The model under review builds one solid part; all positions refer to its coordinate system, in mm. Coordinates: 2 decimals unless noted, no trailing zeros. Order: outer loops, then holes, each group sorted by start corner. A loop starts at its lowest first (then second) coordinate and runs counter-clockwise, first axis right, second up.
from build123d import *

# Parameters (mm, degrees)
SKETCH_1_W      = 20
SKETCH_1_H      = 40
SKETCH_1_R      = 4.5
EXTRUDE_1_DEPTH = 47.5
CHAMFER_1_SIZE  = 2
CHAMFER_2_SIZE  = 2


with BuildPart() as part:
    # 草图1 → 凸台-拉伸1 (new body)
    with BuildSketch(Plane.XY):
        Rectangle(SKETCH_1_W, SKETCH_1_H)
        with Locations((0, 10)):
            Circle(SKETCH_1_R, mode=Mode.SUBTRACT)
        with Locations((0, -10)):
            Circle(SKETCH_1_R, mode=Mode.SUBTRACT)
    extrude(amount=EXTRUDE_1_DEPTH)

    # 倒角1
    chamfer_1_edges = [part.edges().sort_by_distance(p)[0] for p in [
        (-10, -20, 23.75),
    ]]
    chamfer(chamfer_1_edges, length=CHAMFER_1_SIZE)

    # 倒角2
    chamfer_2_edges = [part.edges().sort_by_distance(p)[0] for p in [
        (10, -20, 23.75),
        (-10, 20, 23.75),
        (10, 20, 23.75),
    ]]
    chamfer(chamfer_2_edges, length=CHAMFER_2_SIZE)


solid = part.part
(1) Insertion check: pin 1 Ø7 at (x, y) = (0, -10) entering from +Z. The pin has a flat end and moves straight along its axis. Give the tip position at first contact, or say it passes through.
(2) Consider section A-A (y = -10). Give the boundary of the cut face in (x, z).
(3) Consider section C-C (z = 6.5). Give the boundary of the cut face in (x, y).
(4) Wall thickness on line 1 (Y direction, x = 0, z = 10); line 2 (Y direction, x = 3.5, z = 40.5); line 3 (X direction, y = 14, z = 40.5): over which ranges is each line inside the solid? List them lowest first.
(5) The part is to be moulded in two halves that separate along Y. For faces 1 (the face through (9, -19, 23)), 2 (the face through (-0.98, -14.39, 23.42)), 3 (the face through (0, 0, 0)), 4 (the face through (-0.59, 14.46, 23.42)), say which applies: +Y half, -Y half, draft (parallel to the pull), parting line (faces both ways), or undercut.
(6) Consider section B-B (x = 0). Give the boundary of the cut face in (y, z).
Findings:
1. pin 1: passes through
2. outline: (-10, 0) - (-4.5, 0) - (-4.5, 47.5) - (-10, 47.5) - close; (4.5, 0) - (10, 0) - (10, 47.5) - (4.5, 47.5) - close
3. outline: (-10, -18) - (-8, -20) - (8, -20) - (10, -18) - (10, 18) - (8, 20) - (-8, 20) - (-10, 18) - close; hole circle Ø9 at (0, -10); hole circle Ø9 at (0, 10)
4. line 1: y = -20 to -14.5, -5.5 to 5.5, 14.5 to 20
4. line 2: y = -20 to -12.83, -7.17 to 7.17, 12.83 to 20
4. line 3: x = -10 to -2.06, 2.06 to 10
5. face 1: -Y half
5. face 2: undercut
5. face 3: draft
5. face 4: undercut
6. outline: (-20, 0) - (-14.5, 0) - (-14.5, 47.5) - (-20, 47.5) - close; (-5.5, 0) - (5.5, 0) - (5.5, 47.5) - (-5.5, 47.5) - close; (14.5, 0) - (20, 0) - (20, 47.5) - (14.5, 47.5) - close
